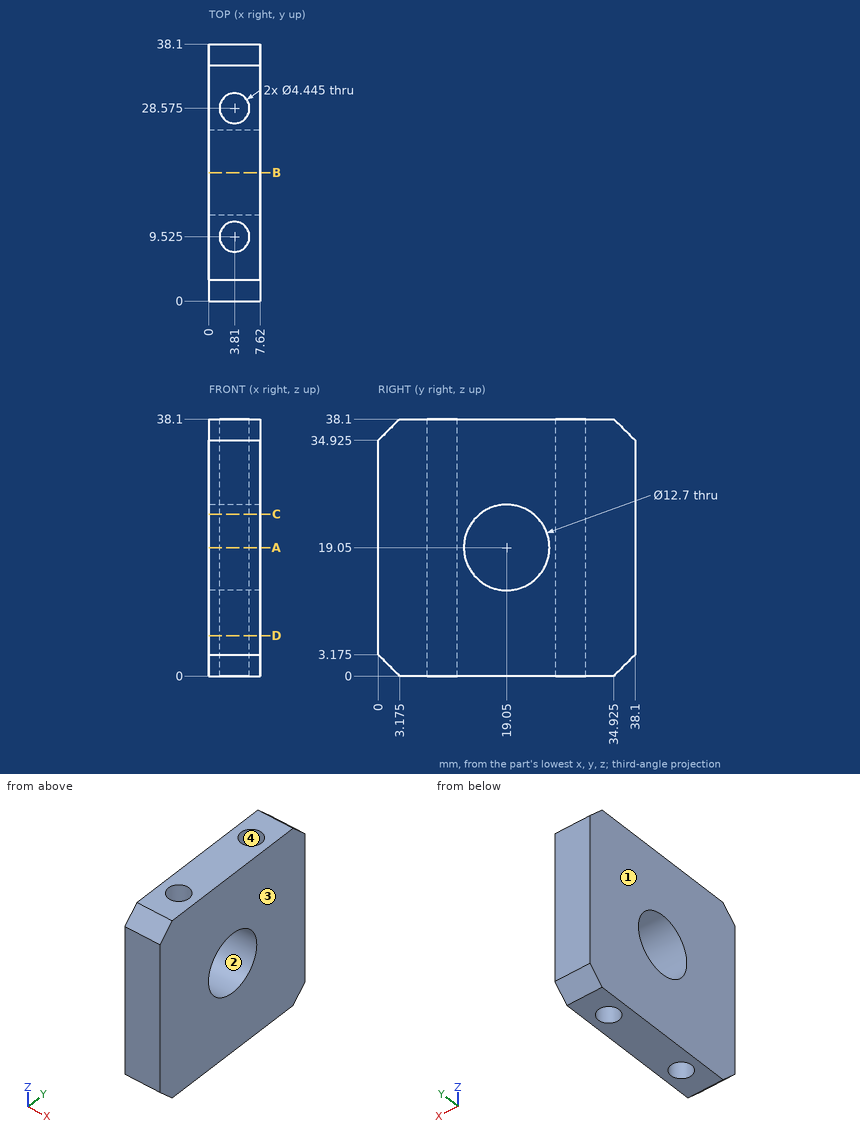
For this review, use the dimensioned drawing (mm, ordinates from the lowest corner) and the shaded views. Coordinates: 2 decimals unless noted, no trailing zeros. Loops run counter-clockwise (first coordinate to the right, second up) from the corner with the lowest first, then second, coordinate; pieces in that order, holes last. Notation, with made-up numbers: (29.25, -19) - (54.25, -19) arc R21 cw to (54.25, -15) - close; hole circle Ø9 at (-5.75, 41.5). An arc over 180 degrees is marked (long way). Use one line per item in the form item = value. Start each with the question number.
1) Take a section at D-D (z = 6). State the section outline as (x, y) points (1 decimal).
2) Draft analysis for pull direction X (two halves, no side actions). For the marked faces 1, 2, 3 and 4, state which applies: released by +X, released by -X, zero draft, split by the parting line, or undercut.
3) For pin 1 (4 mm diameter, centred on x = 3.81, y = 28.575, fed in from -Z), flat-tipped, find the tip position at first contact; note if it passes through.
4) Take a section at C-C (z = 24). State the section outline as (x, y) points (1 decimal), plus the area to 3 significant figures.
5) Take a section at B-B (y = 19.05). State the section outline as (x, z) points, plus the area to 3 significant figures.
6) Take a section at A-A (z = 19.05). State the section outline as (x, y) points (1 decimal), plus the area to 3 significant figures.
7) To check wall thickness, follow probe 1 along Y at (x, z) = (3.81, 9); probe 2 along Z at (x, y) = (4, 19.05); probe 3 along Y at (x, z) = (5.25, 5). State the ranges of each line that lie inside material, in increasing order. Write a range as from..to.
From the geometry:
q1.outline = (0, 0) - (7.6, 0) - (7.6, 38.1) - (0, 38.1) - close; hole circle Ø4.4 at (3.8, 9.5); hole circle Ø4.4 at (3.8, 28.6)
q2.face_1 = released by -X
q2.face_2 = zero draft
q2.face_3 = released by +X
q2.face_4 = undercut
q3.pin_1 = through
q4.outline = (0, 0) - (7.6, 0) - (7.6, 15.1) - (0, 15.1) - close; (0, 23) - (7.6, 23) - (7.6, 38.1) - (0, 38.1) - close; hole circle Ø4.4 at (3.8, 9.5); hole circle Ø4.4 at (3.8, 28.6)
q4.area = 199 mm2
q5.outline = (0, 0) - (7.62, 0) - (7.62, 12.7) - (0, 12.7) - close; (0, 25.4) - (7.62, 25.4) - (7.62, 38.1) - (0, 38.1) - close
q5.area = 194 mm2
q6.outline = (0, 0) - (7.6, 0) - (7.6, 12.7) - (0, 12.7) - close; (0, 25.4) - (7.6, 25.4) - (7.6, 38.1) - (0, 38.1) - close; hole circle Ø4.4 at (3.8, 9.5); hole circle Ø4.4 at (3.8, 28.6)
q6.area = 163 mm2
q7.probe_1 = 0..7.3, 11.75..26.35, 30.8..38.1
q7.probe_2 = 0..12.7, 25.4..38.1
q7.probe_3 = 0..7.83, 11.22..26.88, 30.27..38.1
